from build123d import *

# Parameters (mm, degrees)
EXTRUDE_THIN2_DEPTH     = 19.05
CUT_EXTRUDE1_DEPTH      = 37.122515139
CUT_EXTRUDE1_DEPTH_BACK = 37.122515139
SKETCH7_R               = 5.207
SKETCH7_R_2             = 3.556
CUT_EXTRUDE2_DEPTH      = 37.122515139
CUT_EXTRUDE2_DEPTH_BACK = 37.122515139
SKETCH8_R               = 3.556
FILLET1_R               = 0.79375


with BuildPart() as part:
    # Sketch5 → Extrude-Thin2 (new, symmetric)
    with BuildSketch(Plane(origin=(0, 0, 0), x_dir=(0, 0, -1), z_dir=(1, 0, 0))):
        with BuildLine():
            Line((-27.94, -9.525), (-9.68375, -9.525))
            ThreePointArc((-9.68375, -9.525), (-9.122483992, -9.292516008), (-8.89, -8.73125))
            Line((-8.89, -8.73125), (-8.89, 8.73125))
            ThreePointArc((-8.89, 8.73125), (-7.727580038, 11.537580038), (-4.92125, 12.7))
            Line((-4.92125, 12.7), (27.94, 12.7))
            Line((27.94, 12.7), (27.94, 9.525))
            Line((27.94, 9.525), (-4.92125, 9.525))
            ThreePointArc((-4.92125, 9.525), (-5.482516008, 9.292516008), (-5.715, 8.73125))
            Line((-5.715, 8.73125), (-5.715, -8.73125))
            ThreePointArc((-5.715, -8.73125), (-6.877419962, -11.537580038), (-9.68375, -12.7))
            Line((-9.68375, -12.7), (-27.94, -12.7))
            Line((-27.94, -12.7), (-27.94, -9.525))
        make_face()
    extrude(amount=EXTRUDE_THIN2_DEPTH, both=True)

    # Sketch7 → Cut-Extrude1 (cut, two sides: drawn at the far end of the back side and taken through both)
    with BuildSketch(Plane(origin=(0, 0, 0), x_dir=(1, 0, 0), z_dir=(0, 1, 0)).offset(-CUT_EXTRUDE1_DEPTH_BACK)):
        with Locations(Location((0, 10.414, 0), (0, 0, 270))):
            Circle(SKETCH7_R)
        with Locations(Location((10.795, -19.304, 0), (0, 0, 270))):
            Circle(SKETCH7_R_2)
        with Locations(Location((-10.795, -19.304, 0), (0, 0, 270))):
            Circle(SKETCH7_R_2)
    extrude(amount=CUT_EXTRUDE1_DEPTH + CUT_EXTRUDE1_DEPTH_BACK, mode=Mode.SUBTRACT)

    # Sketch8 → Cut-Extrude2 (cut, two sides: drawn at the far end of the back side and taken through both)
    with BuildSketch(Plane.XY.offset(-CUT_EXTRUDE2_DEPTH_BACK)):
        with Locations((10.795, -0.254)):
            Circle(SKETCH8_R)
        with Locations((-10.795, -0.254)):
            Circle(SKETCH8_R)
    extrude(amount=CUT_EXTRUDE2_DEPTH + CUT_EXTRUDE2_DEPTH_BACK, mode=Mode.SUBTRACT)

    # Fillet1
    fillet1_edges = [part.edges().sort_by_distance(p)[0] for p in [
        (-19.05, -11.1125, 27.94),
        (-19.05, 11.1125, -27.94),
        (19.05, -11.1125, 27.94),
        (19.05, 11.1125, -27.94),
    ]]
    fillet(fillet1_edges, radius=FILLET1_R)


solid = part.part
Can you work these out from the model? Positions are in its coordinate system, mm. A direction names the side the tool comes from. Round coordinates to 2 decimals unless told otherwise and drop trailing zeros. Order: outer loops, then holes, each group sorted by start corner. A loop starts at its lowest first (then second) coordinate and runs counter-clockwise, first axis right, second up. Notation, with made-up numbers: M -34,13 L -9,13 A6 ccw -9,23 Z; hole C 25.25,89 d6. An arc over 180 degrees is marked long. Use a Markdown table: item, result.
1) Imagine slicing it at B-B (x = 12.5). List the corners of the cut face in (y, z) for me (1 decimal).
Geometry says:
| item | result |
|---|---|
| outline | M -12.7,9.7 A4 ccw -8.7,5.7 L -3.4,5.7 L -3.4,8.9 L -8.7,8.9 A0.8 cw -9.5,9.7 L -9.5,16.2 L -12.7,16.2 Z; M -12.7,22.4 L -9.5,22.4 L -9.5,27.9 L -12.7,27.9 Z; M 2.9,5.7 L 8.7,5.7 A0.8 cw 9.5,4.9 L 9.5,-27.9 L 12.7,-27.9 L 12.7,4.9 A4 ccw 8.7,8.9 L 2.9,8.9 Z |
2) If we mould it in two halves opening along X, with no side actions, what happens to faces 4 (the face through (0, -12.7, 19)), 5 (the face through (-19.05, 2, 6)), 6 (the face through (-7.4, 0.8, 7.3))? For each: +X half, -X half, draft (parallel to the pull), parting line (faces both ways), or undercut.
Geometry says:
| item | result |
|---|---|
| face 4 | draft |
| face 5 | -X half |
| face 6 | undercut |
3) I'm going to push flat-ended pins straight in: P1, Ø9, axis at x = -2, z = 20, coming from the +Y side (3 decimals); P2, Ø8, axis at x = -6, y = 7, coming from the -Z side; P3, Ø10, axis at x = -7, z = -13.5, coming from the -Y side (3 decimals); P4, Ø2, axis at x = -5, y = -1.5, coming from the -Z side (3 decimals). Where does each tip first touch, or does it pass through?
Geometry says:
| item | result |
|---|---|
| P1 | stops at y = -9.525 |
| P2 | stops at z = -27.94 |
| P3 | stops at y = 9.525 |
| P4 | stops at z = 5.715 |
4) Imagine slicing it at D-D (z = -10.5). List the corners of the cut face in (x, y) for me (3 decimals).
Geometry says:
| item | result |
|---|---|
| outline | M -19.05,9.525 L -5.206,9.525 L -5.206,12.7 L -19.05,12.7 Z; M 5.206,9.525 L 19.05,9.525 L 19.05,12.7 L 5.206,12.7 Z |
5) Imagine slicing it at A-A (x = 0). List the corners of the cut face in (y, z) for me (1 decimal), then the cut area to 3 significant figures.
Geometry says:
| item | result |
|---|---|
| outline | M -12.7,9.7 A4 ccw -8.7,5.7 L 8.7,5.7 A0.8 cw 9.5,4.9 L 9.5,-5.2 L 12.7,-5.2 L 12.7,4.9 A4 ccw 8.7,8.9 L -8.7,8.9 A0.8 cw -9.5,9.7 L -9.5,27.9 L -12.7,27.9 Z; M 9.5,-27.9 L 12.7,-27.9 L 12.7,-15.6 L 9.5,-15.6 Z |
| area | 208 mm² |
6) On a 3-axis mill with a long thin cutter (end or side, diameter ignored), from which of +Z, -Z, +X, -X, +Y, -Y can I reach the whole of each face in a straight line? I mean faces 1 (the face through (0, 0, 8.89)), 2 (the face through (19.05, 2, 6)), 3 (the face through (5, 9.525, -15)). Say none if no direction works.
Geometry says:
| item | result |
|---|---|
| face 1 | +Z, +X, -X, +Y |
| face 2 | +Z, -Z, +X, +Y, -Y |
| face 3 | -Z, +X, -X, -Y |
7) If I drill on line 1 along Z through (x, y) = (-3, -1.5) (3 decimals); line 2 along Z through (x, y) = (0, 11.5); line 3 along Y through (x, z) = (-14, 3) (3 decimals), over which ranges is the centre line in solid material (lowest first)?
Geometry says:
| item | result |
|---|---|
| line 1 | z = 5.715 to 8.89 |
| line 2 | z = -27.94 to -15.62, -5.21 to 7.76 |
| line 3 | y = 9.525 to 12.7 |
8) Imagine slicing it at C-C (z = 17.5). List the corners of the cut face in (x, y) for me (3 decimals), then the cut area to 3 significant figures.
Geometry says:
| item | result |
|---|---|
| outline | M -19.05,-12.7 L -13.859,-12.7 L -13.859,-9.525 L -19.05,-9.525 Z; M -7.731,-12.7 L 7.731,-12.7 L 7.731,-9.525 L -7.731,-9.525 Z; M 13.859,-12.7 L 19.05,-12.7 L 19.05,-9.525 L 13.859,-9.525 Z |
| area | 82.0 mm² |
